Can you work these out from the model? Positions are in its coordinate system, mm. Give positions to 0.01 mm unless a question says otherwise; leave off trailing zeros. Order: outer loops, then holes, each group sorted by start corner. A loop starts at its lowest first (then second) coordinate and runs counter-clockwise, first axis right, second up. Notation, with made-up numbers: (8, 65.5) -> (25, 65.5) arc R19 cw to (25, 100.5) -> close; hole circle Ø8 at (63.5, 59.5). An arc over 180 degrees is marked (long way). Answer as a JSON object with one key per item and string values.
```python
from build123d import *

# Parameters (mm, degrees)
SKETCH1_W           = 300
SKETCH1_H           = 250
BOSS_EXTRUDE1_DEPTH = 1.25
SKETCH5_W           = 300
SKETCH5_H           = 250
SKETCH5_W_2         = 297.5
SKETCH5_H_2         = 247.5
BOSS_EXTRUDE2_DEPTH = 120
SKETCH6_W           = 300
SKETCH6_H           = 250
BOSS_EXTRUDE3_DEPTH = 1.25


with BuildPart() as part:
    # Sketch1 → Boss-Extrude1 (new body)
    with BuildSketch(Plane(origin=(0, 0, 0), x_dir=(1, 0, 0), z_dir=(0, 1, 0))):
        Rectangle(SKETCH1_W, SKETCH1_H)
    extrude(amount=BOSS_EXTRUDE1_DEPTH)

    # Sketch5 → Boss-Extrude2 (add)
    with BuildSketch(Plane(origin=(0, 0, 0), x_dir=(1, 0, 0), z_dir=(0, 1, 0))):
        Rectangle(SKETCH5_W, SKETCH5_H)
        Rectangle(SKETCH5_W_2, SKETCH5_H_2, mode=Mode.SUBTRACT)
    extrude(amount=BOSS_EXTRUDE2_DEPTH)

    # Sketch6 → Boss-Extrude3 (add)
    with BuildSketch(Plane(origin=(0, 120, 0), x_dir=(1, 0, 0), z_dir=(0, 1, 0))):
        Rectangle(SKETCH6_W, SKETCH6_H)
    extrude(amount=-BOSS_EXTRUDE3_DEPTH)


solid = part.part
```
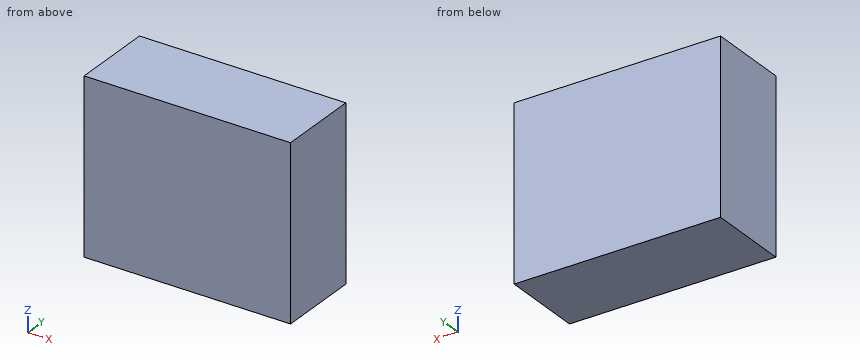
1. Please list where these lines run through material, in increasing order: L1, parallel to Z at x = -23.5, y = 90; L2, parallel to X at y = 60.5, z = 73; L3, parallel to Y at x = 110, z = -92.
Worked answers:
{"L1": "-125 to -123.75, 123.75 to 125", "L2": "-150 to -148.75, 148.75 to 150", "L3": "0 to 1.25, 118.75 to 120"}
2. If we section it at A-A on z = 17.5: Please give me the cut outline in (x, y), then the cut area to 3 significant figures.
Worked answers:
{"outline": "(-150, 0) -> (150, 0) -> (150, 120) -> (-150, 120) -> close; hole (-148.75, 1.25) -> (148.75, 1.25) -> (148.75, 118.75) -> (-148.75, 118.75) -> close", "area": "1,040 mm²"}
3. If we section it at B-B on x = 114.5: Please give me the cut outline in (y, z).
Worked answers:
{"outline": "(0, -125) -> (120, -125) -> (120, 125) -> (0, 125) -> close; hole (1.25, -123.75) -> (118.75, -123.75) -> (118.75, 123.75) -> (1.25, 123.75) -> close"}
